Could you check a few things on this model? Use its own coordinates, in mm. Face numbers are marked on the shaded views. A direction names the side the tool comes from. Coordinates: 2 decimals unless noted, no trailing zeros.
from build123d import *

# Parameters (mm, degrees)
SKETCH_1_RX              = 13.5
SKETCH_1_RY              = 8.5
EXTRUDE_1_DEPTH          = 10
CUT_EXTRUDE_START        = 18.4
SKETCH_2_W               = 5
SKETCH_2_H               = 16.987350845
CUT_EXTRUDE_2_DEPTH      = 10
CUT_EXTRUDE_3_DEPTH      = 24.758998465
CUT_EXTRUDE_3_DEPTH_BACK = 24.758998465
SKETCH_3_R               = 1.9
SKETCH_6_R               = 5
EXTRUDE_3_DEPTH          = 4
CUT_EXTRUDE_5_DEPTH      = 3.2
CHAMFER_1_SIZE           = 1


with BuildPart() as part:
    # ｽｹｯﾁ1 → ﾎﾞｽ - 押し出し1 (new body)
    with BuildSketch(Plane.XY):
        with Locations(Location((0, 0), (0, 0, 180))):
            Ellipse(SKETCH_1_RX, SKETCH_1_RY)
    extrude(amount=EXTRUDE_1_DEPTH)

    # ｽｹｯﾁ2 → ｶｯﾄ - 押し出し2 (cut)
    with BuildSketch(Plane(origin=(0, 0, 0), x_dir=(1, 0, 0), z_dir=(0, 1, 0)).offset(CUT_EXTRUDE_START)):
        with Locations((0, -4.794388707)):
            Rectangle(SKETCH_2_W, SKETCH_2_H)
    cut_extrude_2 = extrude(amount=-CUT_EXTRUDE_2_DEPTH, mode=Mode.SUBTRACT)

    # ﾐﾗｰ1: ｶｯﾄ - 押し出し2 across plane
    add(cut_extrude_2.mirror(Plane.ZX), mode=Mode.SUBTRACT)

    # ｽｹｯﾁ3 → ｶｯﾄ - 押し出し3 (cut, two sides: drawn at the far end of the back side and taken through both)
    with BuildSketch(Plane(origin=(0, 8.4, 0), x_dir=(1, 0, 0), z_dir=(0, 1, 0)).offset(-CUT_EXTRUDE_3_DEPTH_BACK)):
        with Locations(Location((0, -5, 0), (0, 0, 270))):
            Circle(SKETCH_3_R)
    extrude(amount=CUT_EXTRUDE_3_DEPTH + CUT_EXTRUDE_3_DEPTH_BACK, mode=Mode.SUBTRACT)

    # ｽｹｯﾁ6 → ﾎﾞｽ - 押し出し3 (add)
    with BuildSketch(Plane.XY.offset(10)):
        Circle(SKETCH_6_R)
    extrude(amount=EXTRUDE_3_DEPTH)

    # ｽｹｯﾁ5 → ｶｯﾄ - 押し出し5 (cut)
    with BuildSketch(Plane.XY.offset(14)):
        Polygon((-0.05, 2.95), (-0.05, 3.95), (0.05, 3.95), (0.05, 2.95), (0.362514094, 2.637485906), (0.747754611, 2.854095836), (1.017551382, 3.817013124), (1.11384311, 3.790033446), (0.844046339, 2.827116159), (1.060656269, 2.441875642), (1.490051682, 2.546516441), (2.009635632, 3.400935845), (2.095077573, 3.34897745), (1.575493623, 2.494558046), (1.680134421, 2.065162633), (2.121838437, 2.050073571), (2.852674402, 2.732626714), (2.920929716, 2.659543117), (2.190093752, 1.976989974), (2.17500469, 1.535285958), (2.596258142, 1.401586122), (3.484143361, 1.86165116), (3.530149865, 1.772862638), (2.642264646, 1.3127976), (2.50856481, 0.891544148), (2.878125258, 0.649149443), (3.857209346, 0.852605456), (3.877554947, 0.754697047), (2.898470859, 0.551241034), (2.656076155, 0.181680586), (2.94653499, -0.151431681), (3.944203759, -0.219674094), (3.937379518, -0.319440971), (2.939710748, -0.251198558), (2.606598481, -0.541657393), (2.796413701, -0.94078181), (3.738674623, -1.275661422), (3.705186662, -1.369887514), (2.76292574, -1.035007902), (2.363801323, -1.224823122), (2.4388952, -1.660358456), (3.255865093, -2.237038778), (3.198197061, -2.318735767), (2.381227168, -1.742055445), (1.945691834, -1.817149322), (1.900495, -2.25679391), (2.531582945, -3.032505201), (2.454011816, -3.095613995), (1.822923871, -2.319902705), (1.383279283, -2.274705871), (1.22114378, -2.685853285), (1.61954487, -3.603064586), (1.52782374, -3.642904695), (1.12942265, -2.725693394), (0.718275236, -2.563557891), (0.451225912, -2.915715208), (0.587392561, -3.906401154), (0.488323967, -3.920017819), (0.352157318, -2.929331873), (0, -2.66228255), (-0.352157318, -2.929331873), (-0.488323967, -3.920017819), (-0.587392561, -3.906401154), (-0.451225912, -2.915715208), (-0.718275236, -2.563557891), (-1.12942265, -2.725693394), (-1.52782374, -3.642904695), (-1.61954487, -3.603064586), (-1.22114378, -2.685853285), (-1.383279283, -2.274705871), (-1.822923871, -2.319902705), (-2.454011816, -3.095613995), (-2.531582945, -3.032505201), (-1.900495, -2.25679391), (-1.945691834, -1.817149322), (-2.381227168, -1.742055445), (-3.198197061, -2.318735767), (-3.255865093, -2.237038778), (-2.4388952, -1.660358456), (-2.363801323, -1.224823122), (-2.76292574, -1.035007902), (-3.705186662, -1.369887514), (-3.738674623, -1.275661422), (-2.796413701, -0.94078181), (-2.606598481, -0.541657393), (-2.939710748, -0.251198558), (-3.937379518, -0.319440971), (-3.944203759, -0.219674094), (-2.94653499, -0.151431681), (-2.656076155, 0.181680586), (-2.898470859, 0.551241034), (-3.877554947, 0.754697047), (-3.857209346, 0.852605456), (-2.878125258, 0.649149443), (-2.50856481, 0.891544148), (-2.642264646, 1.3127976), (-3.530149865, 1.772862638), (-3.484143361, 1.86165116), (-2.596258142, 1.401586122), (-2.17500469, 1.535285958), (-2.190093752, 1.976989974), (-2.920929716, 2.659543117), (-2.852674402, 2.732626714), (-2.121838437, 2.050073571), (-1.680134421, 2.065162633), (-1.575493623, 2.494558046), (-2.095077573, 3.34897745), (-2.009635632, 3.400935845), (-1.490051682, 2.546516441), (-1.060656269, 2.441875642), (-0.844046339, 2.827116159), (-1.11384311, 3.790033446), (-1.017551382, 3.817013124), (-0.747754611, 2.854095836), (-0.362514094, 2.637485906), align=None)
    extrude(amount=-CUT_EXTRUDE_5_DEPTH, mode=Mode.SUBTRACT)

    # 面取り1
    chamfer_1_edges = [part.edges().sort_by_distance(p)[0] for p in [
        (-5, 0, 10),
    ]]
    chamfer(chamfer_1_edges, length=CHAMFER_1_SIZE)


solid = part.part
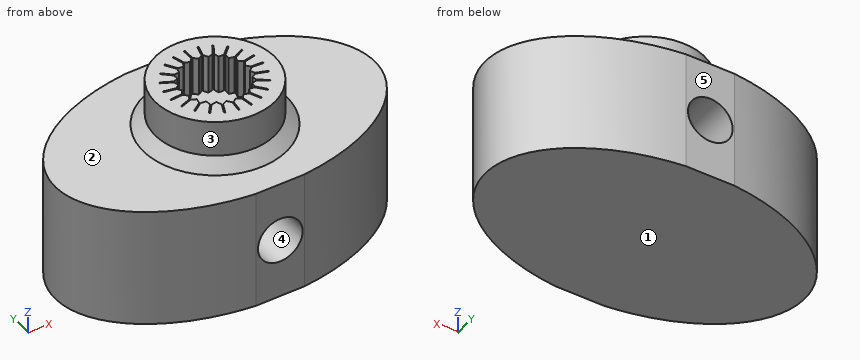
(1) For pin 1 (1.1 mm diameter, centred on y = 3.5, z = 12, fed in from -X); pin 2 (3 mm diameter, centred on x = 0, z = 5, fed in from -Y); pin 3 (2 mm diameter, centred on y = -6.5, z = 2.5, fed in from +X); pin 4 (6 mm diameter, centred on x = 7.5, z = 6, fed in from +Y), each with a flat end and sliding along its axis, tell me the tip position at first contact or that it passes through.
Answers:
pin 1: stops at x = -4.04
pin 2: passes through
pin 3: stops at x = 10.29
pin 4: stops at y = 8.01
(2) Which directions (+Z, -Z, +X, -X, +Y, -Y) give clear straight access to the entire face, cutting with the end or side of a thin tool? Please do the marked faces 1 and 2.
Answers:
face 1: -Z, +X, -X, +Y, -Y
face 2: +Z
(3) We'd pull the mould along X, two halves only. Please class the marked faces 3, 4 and 5: +X half, -X half, draft (parallel to the pull), parting line (faces both ways), or undercut.
Answers:
face 3: parting line
face 4: undercut
face 5: draft
(4) I need wall thicknesses on probe 1 along Z at (x, y) = (0, -1.5); probe 2 along Z at (x, y) = (4, 6.5); probe 3 along X at (y, z) = (-0.5, 12). Which ranges of each line are inside material? Lowest first, please.
Answers:
probe 1: z = 0 to 3.1, 6.9 to 10.8
probe 2: z = 0 to 10
probe 3: x = -4.97 to -2.65, 2.65 to 4.97
